Print and shaded views of the part. All mm, measured from the part's lowest x, y and z. Round coordinates to 2 decimals unless told otherwise and drop trailing zeros. Loops run counter-clockwise (first coordinate to the right, second up) from the corner with the lowest first, then second, coordinate; pieces in that order, holes last. Notation, with made-up numbers: (-38.75, -32.5) - (-34.75, -32.5) arc R27 cw to (-34.75, -4.5) - close; hole circle Ø6 at (57.5, -8.5). An arc over 180 degrees is marked (long way). Use one line per item in the form item = value. Start each with the question number.
Q1. Saw through at A-A (z = 1.6). Count the separate pieces of the cut face and the enclosed holes in it, then the cut area to 3 significant figures.
Q2. Pin check, flat tips, straight feed: pin 1 (4.5 mm diameter, centred on x = 57, y = 15, fed in from +Z); pin 2 (2.5 mm diameter, centred on x = 153.5, z = 3.5, fed in from -Y); pin 3 (2 mm diameter, centred on x = 38, z = 4, fed in from -Y); pin 4 (3 mm diameter, centred on x = 213, z = 2.5, fed in from +Y). Stop position of each tip, or through.
Q3. Saw through at C-C (y = 186.5). Give the cut face in (x, z), then the cut area to 3 significant figures.
Q4. Drill centre lines: line 1 (Y direction, x = 57, z = 1.3); line 2 (X direction, y = 105, z = 1.6); line 3 (Y direction, x = 261, z = 3.4). Where is each one in solid material? Low to high.
Q5. Saw through at B-B (x = 198). Give the cut face in (y, z).
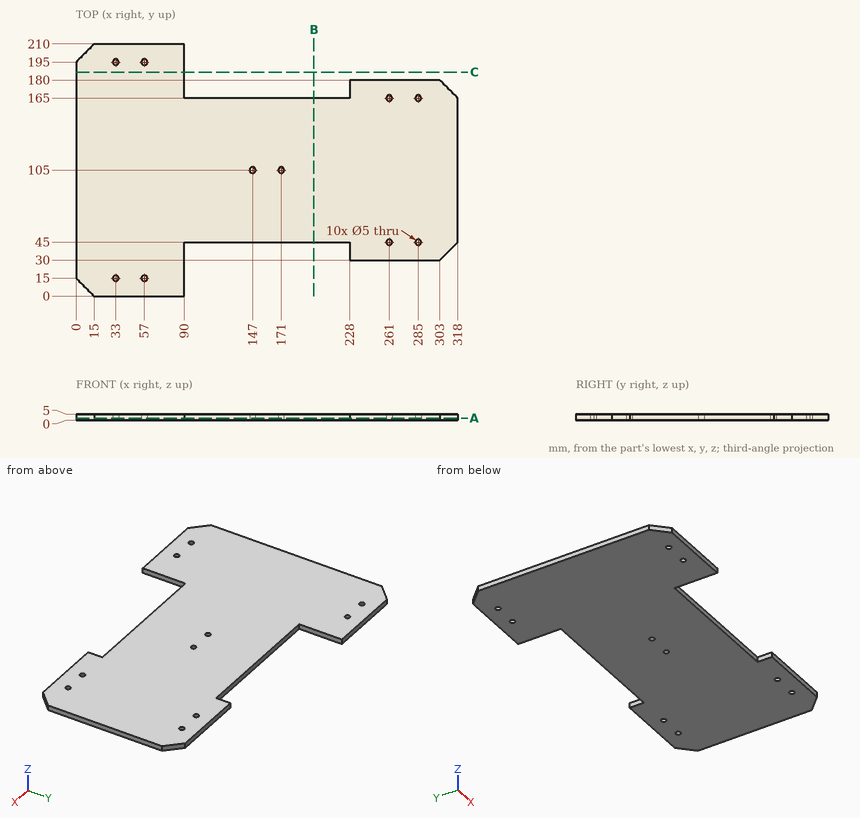
Report:
q1.separate_pieces = 1
q1.enclosed_holes = 10
q1.area = 48,300 mm²
q2.pin_1 = through
q2.pin_2 = 45
q2.pin_3 = 0
q2.pin_4 = 165
q3.outline = (0, 0) - (90, 0) - (90, 5) - (0, 5) - close
q3.area = 450 mm²
q4.line_1 = 0 to 12.5, 17.5 to 192.5, 197.5 to 210
q4.line_2 = 0 to 144.5, 149.5 to 168.5, 173.5 to 318
q4.line_3 = 30 to 42.5, 47.5 to 162.5, 167.5 to 180
q5.outline = (45, 0) - (165, 0) - (165, 5) - (45, 5) - close
